Drawing for the job (mm, zero at the part's lowest x, y, z). A direction names the side the tool comes from. Coordinates: 2 decimals unless noted, no trailing zeros. Write each loop counter-clockwise with the first axis right and the second up, starting at its lowest first coordinate (ties: lowest second). Pieces come first, ordered by that corner, then holes. Notation, with made-up numbers: (-11.5, 87.25) -> (19.5, 87.25) arc R8 cw to (19.5, 96.25) -> close; hole circle Ø9 at (10, 60). An arc over 180 degrees is marked (long way). Answer as CSV lines item,"result".
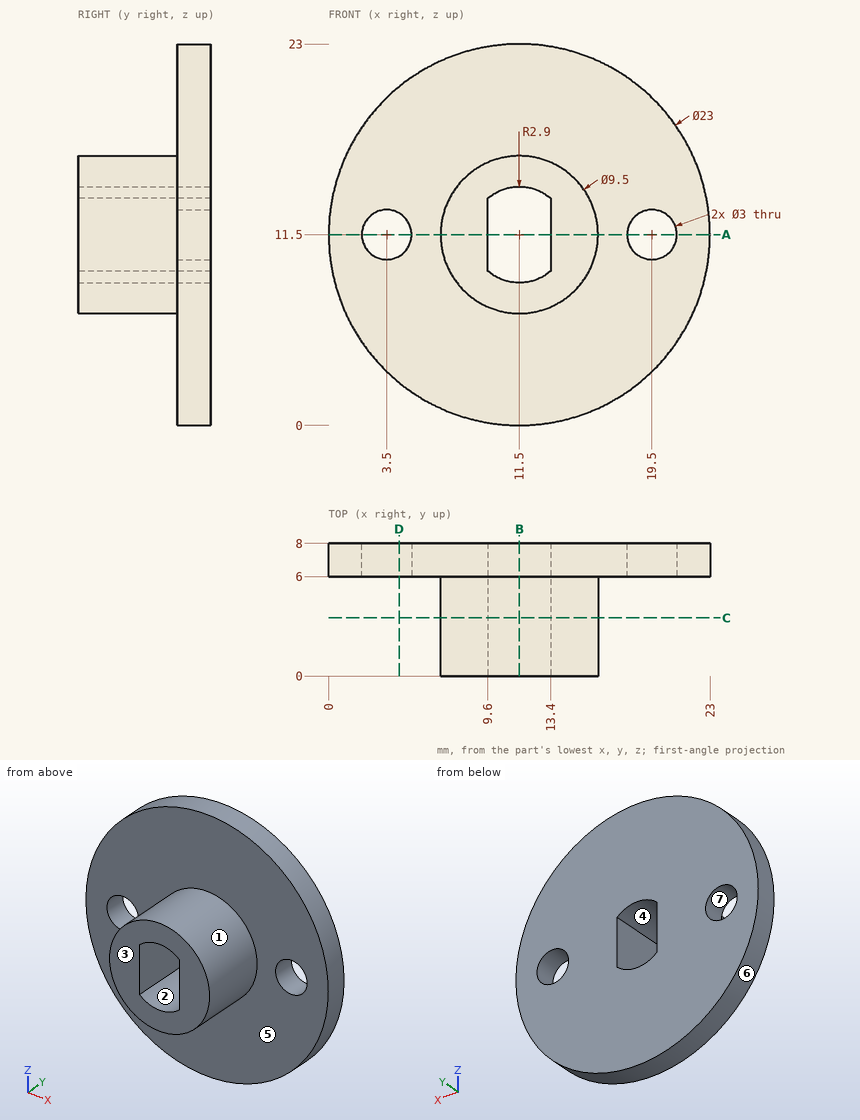
Item 1: Saw through at B-B on x = 11.5. Give the cut face in (y, z), and give its area (3 significant figures).
Answer below:
outline,"(0, 6.75) -> (6, 6.75) -> (6, 0) -> (8, 0) -> (8, 8.6) -> (0, 8.6) -> close; (0, 14.4) -> (8, 14.4) -> (8, 23) -> (6, 23) -> (6, 16.25) -> (0, 16.25) -> close"
area,"56.6 mm2"
Item 2: Saw through at A-A on z = 11.5. Give the cut face in (x, y).
Answer below:
outline,"(0, 6) -> (2, 6) -> (2, 8) -> (0, 8) -> close; (5, 6) -> (6.75, 6) -> (6.75, 0) -> (9.6, 0) -> (9.6, 8) -> (5, 8) -> close; (13.4, 0) -> (16.25, 0) -> (16.25, 6) -> (18, 6) -> (18, 8) -> (13.4, 8) -> close; (21, 6) -> (23, 6) -> (23, 8) -> (21, 8) -> close"
Item 3: Two-plate mould, pull along Z, no slides. Class the marked faces 4, 5, 6 and 7: pulls with the +Z half, pulls with the -Z half, needs draft (parallel to the pull), parting line crosses it, or undercut.
Answer below:
face 4,"undercut"
face 5,"needs draft"
face 6,"parting line crosses it"
face 7,"undercut"
Item 4: Saw through at C-C on y = 3.5. Give the cut face in (x, z), and give its area (3 significant figures).
Answer below:
outline,"circle Ø9.5 at (11.5, 11.5); hole (9.6, 9.31) arc R2.9 ccw to (13.4, 9.31) -> (13.4, 13.69) arc R2.9 ccw to (9.6, 13.69) -> close"
area,"50.5 mm2"
Item 5: Wall check: line 1 (X direction, y = 2, z = 11.25); line 2 (Y direction, x = 5.75, z = 21); line 3 (Z direction, x = 19.5, y = 7). Give the ranges that are in metal, low to high. Write a range as from..to.
Answer below:
line 1,"x = 6.76..9.6, 13.4..16.24"
line 2,"y = 6..8"
line 3,"z = 3.24..10, 13..19.76"
Item 6: 3-axis set-ups, long thin cutter, end or side, ignore diameter. For the marked faces 1, 2 and 3: which of +Z, -Z, +X, -X, +Y, -Y reach the whole face in a straight line?
Answer below:
face 1,"-Y"
face 2,"+Y, -Y"
face 3,"+Z, -Z, +X, -X, -Y"
Item 7: Saw through at D-D on x = 4.25. Give the cut face in (y, z).
Answer below:
outline,"(6, 2.57) -> (8, 2.57) -> (8, 10.2) -> (6, 10.2) -> close; (6, 12.8) -> (8, 12.8) -> (8, 20.43) -> (6, 20.43) -> close"
Item 8: Flat gauge pins, fed straight in: pin 1 (2 mm diameter, centred on x = 4.5, z = 17.5, fed in from -Y); pin 2 (1.8 mm diameter, centred on x = 19.5, z = 11.5, fed in from +Y); pin 3 (1.5 mm diameter, centred on y = 5.5, z = 15, fed in from +X); pin 4 (3.5 mm diameter, centred on y = 2, z = 12.5, fed in from -X). Where does each tip first touch, or does it go through?
Answer below:
pin 1,"stops at y = 6"
pin 2,"passes through"
pin 3,"stops at x = 22.62"
pin 4,"stops at x = 6.75"
